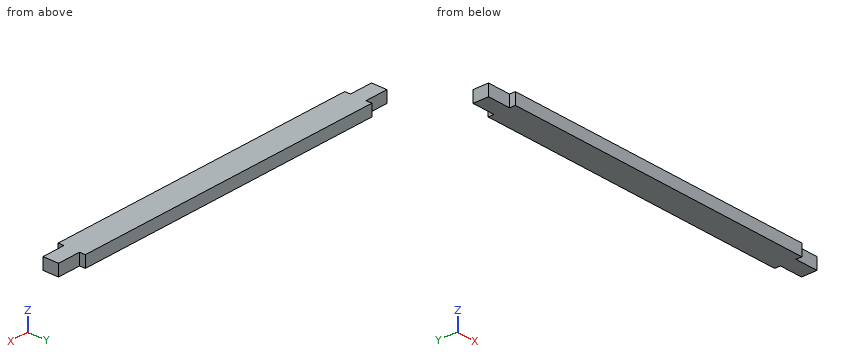
from build123d import *

# Parameters (mm, degrees)
F0_W     = 88.9
F0_H     = 38.1
F1_DEPTH = 1041.4
F2_W     = 50.8
F2_H     = 38.1
F3_DEPTH = 76.2
F4_W     = 50.8
F4_H     = 38.1
F5_DEPTH = 76.2


with BuildPart() as f1:
    # F0 (on Right) → F1 (new body)
    with BuildSketch(Plane.YZ):
        with Locations((44.45, 19.05)):
            Rectangle(F0_W, F0_H)
    extrude(amount=-F1_DEPTH)

    # F2 (on face) → F3 (join)
    with BuildSketch(Plane.YZ):
        with Locations((44.45, 19.05)):
            Rectangle(F2_W, F2_H)
    extrude(amount=F3_DEPTH)

    # F4 (on face) → F5 (join)
    with BuildSketch(Plane(origin=(-1041.4, 0, 0), x_dir=(0, -1, 0), z_dir=(-1, 0, 0))):
        with Locations((-44.45, 19.05)):
            Rectangle(F4_W, F4_H)
    extrude(amount=F5_DEPTH)


solid = f1.part
Geometry: final body of the model. Coordinates: model frame, mm. Give positions to 0.01 mm unless a question says otherwise; leave off trailing zeros. Order: outer loops, then holes, each group sorted by start corner. A loop starts at its lowest first (then second) coordinate and runs counter-clockwise, first axis right, second up. Notation, with made-up numbers: (20.25, 34) -> (69.25, 34) arc R10 ccw to (69.25, 39) -> close; hole circle Ø1 at (45.25, -11). An arc over 180 degrees is marked (long way). Write each question's results on one line, items separated by ' | '.
1) First-contact query: pin 1 Ø15 at (y, z) = (79, 20) entering from -X; pin 2 Ø21 at (y, z) = (11, 10.5) entering from -X; pin 3 Ø11.5 at (x, z) = (22, 19) entering from -Y; pin 4 Ø15 at (y, z) = (81.5, 18.5) entering from +X. Flat tips, straight axial feed; report the tip coordinate or a pass-through.
Geometry says:
pin 1: stops at x = -1041.4 | pin 2: stops at x = -1117.6 | pin 3: stops at y = 19.05 | pin 4: stops at x = 0
2) Cut plane A-A (z = 29). Output: boundary loops of the cut face in (x, y).
Geometry says:
outline: (-1117.6, 19.05) -> (-1041.4, 19.05) -> (-1041.4, 0) -> (0, 0) -> (0, 19.05) -> (76.2, 19.05) -> (76.2, 69.85) -> (0, 69.85) -> (0, 88.9) -> (-1041.4, 88.9) -> (-1041.4, 69.85) -> (-1117.6, 69.85) -> close
3) Line query: line 1 along X through (y, z) = (82.5, 11); line 2 along Y through (x, z) = (1.5, 32). Output: solid intervals per line, ascending.
Geometry says:
line 1: x = -1041.4 to 0 | line 2: y = 19.05 to 69.85
